For this review, take the finished solid that the model builds, in its own axes (mm). A direction names the side the tool comes from. Coordinates: 2 decimals unless noted, no trailing zeros. Loops run counter-clockwise (first coordinate to the right, second up) from the corner with the lowest first, then second, coordinate; pieces in that order, holes last. Notation, with made-up numbers: (3, 28.5) -> (33, 28.5) arc R31 cw to (33, 63.5) -> close; hole circle Ø1 at (10, -10.5). An arc over 180 degrees is marked (long way). Answer in a Markdown table with one row per item.
from build123d import *

# Parameters (mm, degrees)
SKETCH1_W                = 100
SKETCH1_H                = 45
BASE_FLANGE1_DEPTH       = 5
EDGE_FLANGE1_DEPTH       = 100
EDGE_FLANGE2_DEPTH       = 100
EDGE_FLANGE3_DEPTH       = 100
CUT_EXTRUDE1_REACH       = 135.401
SKETCH15_R               = 2.5
CUT_EXTRUDE2_DEPTH       = 10
M5_CLEARANCE_HOLE1_D     = 5.5
M5_CLEARANCE_HOLE1_DEPTH = 15.966
M5_CLEARANCE_HOLE1_TIP   = 1.652366702
BREAK_CORNER1_START      = -52.832474919
BREAK_CORNER1_DEPTH      = 5
BREAK_CORNER1_2_DEPTH    = 5


# Read off the part's stored shape, not the designer's step: Break-Corner1
# Sheet-metal steps are written as plain solids
with BuildPart() as part:
    # Sketch1 → Base-Flange1 (new body)
    with BuildSketch(Plane.XY):
        with Locations((50, 22.5)):
            Rectangle(SKETCH1_W, SKETCH1_H)
    extrude(amount=BASE_FLANGE1_DEPTH)

    # Edge-Flange1 section (across the edge) → Edge-Flange1 (add)
    with BuildSketch(Plane(origin=(100, -0.466307658, 0), x_dir=(0, 0.7660444431189746, -0.6427876096865435), z_dir=(-1, 0, 0))):
        with BuildLine():
            Line((-5, 0.466307658), (-5, 20))
            Line((-5, 20), (0, 20))
            Line((0, 20), (0, 0.466307658))
            ThreePointArc((0, 0.466307658), (0.093692213, 0.043689396), (0.35721239, -0.299736785))
            Line((0.35721239, -0.299736785), (-2.856725658, -4.129959001))
            ThreePointArc((-2.856725658, -4.129959001), (-4.437846722, -2.069401912), (-5, 0.466307658))
        make_face()
    extrude(amount=EDGE_FLANGE1_DEPTH)

    # Edge-Flange2 section (across the edge) → Edge-Flange2 (add)
    with BuildSketch(Plane(origin=(100, -13.556015409, -15.599706238), x_dir=(0, 1, 0), z_dir=(-1, 0, 0))):
        with BuildLine():
            Line((-5, 0.363970234), (-5, 35))
            Line((-5, 35), (0, 35))
            Line((0, 35), (0, 0.363970234))
            ThreePointArc((0, 0.363970234), (0.060307379, 0.021950091), (0.233955557, -0.278817375))
            Line((0.233955557, -0.278817375), (-3.596266659, -3.492755424))
            ThreePointArc((-3.596266659, -3.492755424), (-4.638155725, -1.688150626), (-5, 0.363970234))
        make_face()
    extrude(amount=EDGE_FLANGE2_DEPTH)

    # Edge-Flange3 section (across the edge) → Edge-Flange3 (add)
    with BuildSketch(Plane(origin=(100, -13.556015409, -51.066013896), x_dir=(0, 0.6427876096865516, 0.7660444431189678), z_dir=(-1, 0, 0))):
        with BuildLine():
            Line((-5, 0.466307658), (-5, 25))
            Line((-5, 25), (0, 25))
            Line((0, 25), (0, 0.466307658))
            ThreePointArc((0, 0.466307658), (0.093692213, 0.043689396), (0.35721239, -0.299736785))
            Line((0.35721239, -0.299736785), (-2.856725658, -4.129959001))
            ThreePointArc((-2.856725658, -4.129959001), (-4.437846722, -2.069401912), (-5, 0.466307658))
        make_face()
    extrude(amount=EDGE_FLANGE3_DEPTH)

    # Sketch15 → Cut-Extrude1 (cut, up to next)
    with BuildSketch(Plane.XY.offset(5), mode=Mode.PRIVATE) as cut_extrude1_sk1:
        with Locations((80, 5)):
            Circle(SKETCH15_R)
    cut_extrude1_tool1 = extrude(cut_extrude1_sk1.sketch, amount=-CUT_EXTRUDE1_REACH, mode=Mode.PRIVATE) & part.part
    # Sketch15 → Cut-Extrude1 (cut, up to next)
    with BuildSketch(Plane.XY.offset(5), mode=Mode.PRIVATE) as cut_extrude1_sk2:
        with Locations((80, 25)):
            Circle(SKETCH15_R)
    cut_extrude1_tool2 = extrude(cut_extrude1_sk2.sketch, amount=-CUT_EXTRUDE1_REACH, mode=Mode.PRIVATE) & part.part
    # Sketch15 → Cut-Extrude1 (cut, up to next)
    with BuildSketch(Plane.XY.offset(5), mode=Mode.PRIVATE) as cut_extrude1_sk3:
        with BuildLine():
            Line((10, 40), (25, 40))
            ThreePointArc((25, 40), (28, 37), (25, 34))
            Line((25, 34), (10, 34))
            ThreePointArc((10, 34), (7, 37), (10, 40))
        make_face()
    cut_extrude1_tool3 = extrude(cut_extrude1_sk3.sketch, amount=-CUT_EXTRUDE1_REACH, mode=Mode.PRIVATE) & part.part
    # Sketch15 → Cut-Extrude1 (cut, up to next)
    with BuildSketch(Plane.XY.offset(5), mode=Mode.PRIVATE) as cut_extrude1_sk4:
        with BuildLine():
            Line((75, 40), (90, 40))
            ThreePointArc((90, 40), (93, 37), (90, 34))
            Line((90, 34), (75, 34))
            ThreePointArc((75, 34), (72, 37), (75, 40))
        make_face()
    cut_extrude1_tool4 = extrude(cut_extrude1_sk4.sketch, amount=-CUT_EXTRUDE1_REACH, mode=Mode.PRIVATE) & part.part
    add(cut_extrude1_tool1.solids().sort_by_distance((80, 5, 5))[0], mode=Mode.SUBTRACT)
    add(cut_extrude1_tool2.solids().sort_by_distance((80, 25, 5))[0], mode=Mode.SUBTRACT)
    add(cut_extrude1_tool3.solids().sort_by_distance((17.5, 37, 5))[0], mode=Mode.SUBTRACT)
    add(cut_extrude1_tool4.solids().sort_by_distance((82.5, 37, 5))[0], mode=Mode.SUBTRACT)

    # Sketch16 → Cut-Extrude2 (cut)
    with BuildSketch(Plane(origin=(0, -30.746122218, -36.641801612), x_dir=(1, 0, 0), z_dir=(0, 0.6427876096865515, 0.7660444431189678))):
        with BuildLine():
            Line((10, 42.440090734), (25, 42.440090734))
            ThreePointArc((25, 42.440090734), (28, 39.440090734), (25, 36.440090734))
            Line((25, 36.440090734), (10, 36.440090734))
            ThreePointArc((10, 36.440090734), (7, 39.440090734), (10, 42.440090734))
        make_face()
        with BuildLine():
            Line((75, 42.440090734), (90, 42.440090734))
            ThreePointArc((90, 42.440090734), (93, 39.440090734), (90, 36.440090734))
            Line((90, 36.440090734), (75, 36.440090734))
            ThreePointArc((75, 36.440090734), (72, 39.440090734), (75, 42.440090734))
        make_face()
    extrude(amount=-CUT_EXTRUDE2_DEPTH, mode=Mode.SUBTRACT)

    # M5 Clearance Hole1
    with Locations(Plane.XY.offset(5)):
        with Locations((80, 25), (80, 5)):
            Hole(M5_CLEARANCE_HOLE1_D / 2, depth=M5_CLEARANCE_HOLE1_DEPTH)
            with Locations((0, 0, -(M5_CLEARANCE_HOLE1_DEPTH + M5_CLEARANCE_HOLE1_TIP / 2))):  # 118° drill point
                Cone(0, M5_CLEARANCE_HOLE1_D / 2, M5_CLEARANCE_HOLE1_TIP, mode=Mode.SUBTRACT)

    # Break-Corner1 outline → Break-Corner1 (cut)
    with BuildSketch(Plane(origin=(0, 0, 0), x_dir=(1, 0, 0), z_dir=(0, 0.6427876096865517, 0.7660444431189677)).offset(BREAK_CORNER1_START)):
        with BuildLine():
            ThreePointArc((0, 42.440090734), (1.464466094, 45.97562464), (5, 47.440090734))
            Line((5, 47.440090734), (0, 47.440090734))
            Line((0, 47.440090734), (0, 42.440090734))
        make_face()
        with BuildLine():
            ThreePointArc((95, 47.440090734), (98.535533906, 45.97562464), (100, 42.440090734))
            Line((100, 42.440090734), (100, 47.440090734))
            Line((100, 47.440090734), (95, 47.440090734))
        make_face()
    extrude(amount=BREAK_CORNER1_DEPTH, mode=Mode.SUBTRACT)

    # Break-Corner1 2 outline → Break-Corner1 2 (cut)
    with BuildSketch(Plane.XY):
        with BuildLine():
            Line((0, 45), (0, 40))
            ThreePointArc((0, 40), (1.464466094, 43.535533906), (5, 45))
            Line((5, 45), (0, 45))
        make_face()
        with BuildLine():
            Line((100, 45), (95, 45))
            ThreePointArc((95, 45), (98.535533906, 43.535533906), (100, 40))
            Line((100, 40), (100, 45))
        make_face()
    extrude(amount=BREAK_CORNER1_2_DEPTH, mode=Mode.SUBTRACT)


solid = part.part
Item 1: Take a section at D-D, the plane x = 32. State the section outline as (y, z) points, and give its area (3 significant figures).
Worked answers:
| item | result |
|---|---|
| outline | (-18.56, -50.6) arc R6 ccw to (-16.41, -55.2) -> (2.38, -70.97) -> (5.6, -67.14) -> (-13.2, -51.37) arc R1 cw to (-13.56, -50.6) -> (-13.56, -15.96) arc R1 cw to (-13.32, -15.32) -> (-0.77, -0.36) arc R1 cw to (0, 0) -> (45, 0) -> (45, 5) -> (0, 5) arc R6 ccw to (-4.6, 2.86) -> (-17.15, -12.11) arc R6 ccw to (-18.56, -15.96) -> close |
| area | 661 mm² |
Item 2: Take a section at C-C, the plane y = -8. State the section outline as (x, z) points.
Worked answers:
| item | result |
|---|---|
| outline | (0, -62.26) -> (100, -62.26) -> (100, -55.73) -> (0, -55.73) -> close; (0, -8.98) -> (100, -8.98) -> (100, -1.2) -> (0, -1.2) -> close |
Item 3: Take a section at A-A, the plane x = 84.5. State the section outline as (y, z) points.
Worked answers:
| item | result |
|---|---|
| outline | (-18.56, -50.6) arc R6 ccw to (-16.41, -55.2) -> (-6.05, -63.9) -> (-2.83, -60.07) -> (-13.2, -51.37) arc R1 cw to (-13.56, -50.6) -> (-13.56, -15.96) arc R1 cw to (-13.32, -15.32) -> (-0.77, -0.36) arc R1 cw to (0, 0) -> (34, 0) -> (34, 5) -> (0, 5) arc R6 ccw to (-4.6, 2.86) -> (-17.15, -12.11) arc R6 ccw to (-18.56, -15.96) -> close; (-1.45, -67.75) -> (2.38, -70.97) -> (5.6, -67.14) -> (1.76, -63.92) -> close; (40, 0) -> (45, 0) -> (45, 5) -> (40, 5) -> close |
Item 4: Take a section at B-B, the plane y = 37. State the section outline as (x, z) points, and give its area (3 significant figures).
Worked answers:
| item | result |
|---|---|
| outline | (0, 0) -> (7, 0) -> (7, 5) -> (0, 5) -> close; (28, 0) -> (72, 0) -> (72, 5) -> (28, 5) -> close; (93, 0) -> (100, 0) -> (100, 5) -> (93, 5) -> close |
| area | 290 mm² |
Item 5: For L1, parallel to Y at x = 80, z = 1.5; L2, parallel to Y at x = 80, z = 1; L3, parallel to Z at x = 87.5, y = 30, list the stretches that pass through material, from the lowest coordinate up.
Worked answers:
| item | result |
|---|---|
| L1 | -5.73 to 2.25, 7.75 to 22.25, 27.75 to 34, 40 to 45 |
| L2 | -6.15 to 2.25, 7.75 to 22.25, 27.75 to 34, 40 to 45 |
| L3 | 0 to 5 |
Item 6: For faces 4 (the cylindrical face through (7, -2.17, -63.84)), 5 (the flat face through (100, -14, -23)), 6 (the flat face through (17.605, -4.416, -61.953)), 7 (the flat face through (82, 40, 3)), list the 3-axis set-ups (+Z, -Z, +X, -X, +Y, -Y) from which the entire face can be reached by the end or side of a thin tool; tool diameter is ignored.
Worked answers:
| item | result |
|---|---|
| face 4 | none |
| face 5 | +Z, -Z, +X, +Y, -Y |
| face 6 | -Z, +Y |
| face 7 | +Z, -Z |
Item 7: Insertion check: pin 1 (2 mm diameter, centred on x = 85, z = -26.5, fed in from +Y); pin 2 (1.5 mm diameter, centred on x = 86, z = 2, fed in from -Y); pin 3 (13.5 mm diameter, centred on x = 46.5, y = 22, fed in from -Z). Each pin has a flat end and moves straight along its axis. Give the tip position at first contact, or say it passes through.
Worked answers:
| item | result |
|---|---|
| pin 1 | y = -13.56 |
| pin 2 | y = -5.94 |
| pin 3 | z = 0 |
Item 8: The part is to be moulded in two halves that separate along Z. For faces 1 (the cylindrical face through (93, -2.1, -63.9)), 2 (the cylindrical face through (50.7, -18.184, -13.884)), 3 (the cylindrical face through (7, 37, 3)), say which applies: +Z half, -Z half, draft (parallel to the pull), parting line (faces both ways), or undercut.
Worked answers:
| item | result |
|---|---|
| face 1 | undercut |
| face 2 | +Z half |
| face 3 | draft |
